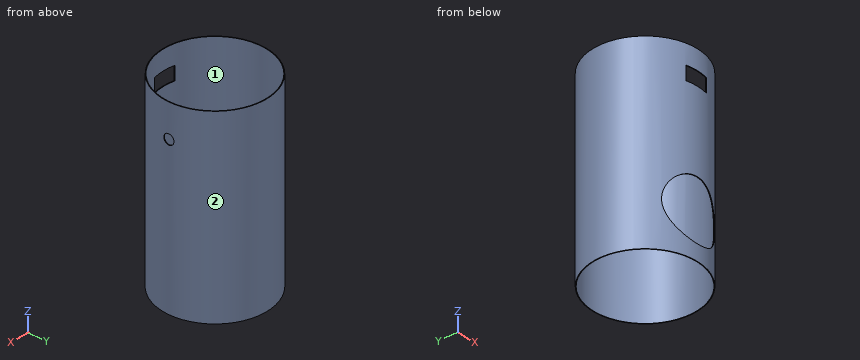
Autodesk Inventor part; units mm, degrees
ref_plane "WeldJoint" through (0, 0, -10) normal (0.5299, -0.848, 0) x (0, 0, 1)
ref_plane "Outer" through (0, 0, -10) normal (0.454, -0.891, 0) x (0, 0, 1)
ref_plane "Clock_Feeder" through (0, 0, -10) normal (0, 1, 0) x (0, 0, 1)
sketch "Sketch13" plane through (0, 0, 0) normal (0, 0, 1) x (1, 0, 0)
  circle A0 centre (0, 0) radius 470 construction
  line L0 (0, 0) -> (0, -470)
  line L1 (0, 0) -> (-398.5826, -249.0621)
  line L2 (0, 0) -> (470, 0)
  line L3 (0, 0) -> (0, -470)
  line L4 (0, 0) -> (0, -470)
  line L5 (0, 0) -> (-418.7731, -213.3755)
  arc A1 (-398.5826, -249.0621) -> (0, -470) centre (0, 0) ccw
  dimension "d53" = 940
  dimension "d54" = 58
  dimension "d55" = 0
  dimension "d56" = 0
  dimension "d57" = 270
  dimension "d58" = 63
ref_plane "WeldJoint" through (0, 0, -10) normal (0.5299, -0.848, 0) x (0, 0, 1)
ref_plane "Outer" through (0, 0, -10) normal (0.454, -0.891, 0) x (0, 0, 1)
ref_plane "Clock_Feeder" through (0, 0, -10) normal (0, 1, 0) x (0, 0, 1)
ref_plane "Charging" through (0, 0, -10) normal (1, 0, 0) x (0, 0, 1)
ref_plane "Accsess" through (0, 0, -10) normal (1, 0, 0) x (0, 0, 1)
sketch "Sketch14" plane through (0, 0, -10) normal (0.5299, -0.848, 0) x (0, 0, 1)
  line L0 (1710, 464) -> (10, 464)
  line L1 (10, 464) -> (10, 470)
  line L2 (10, 470) -> (1710, 470)
  line L3 (1710, 470) -> (1710, 464)
  line L4 (10, 0) -> (825.0673, 0)
  point P0 (10, 467)
  dimension "d59" = 1700
  dimension "d60" = 6
  dimension "d61" = 940
revolve "Revolution2" add sketch "Sketch14" angle 359.9 about axis through (0, 0, 0) along (0, 0, 1)
sketch "Sketch AnglePlane_Feeder" plane through (0, 0, -10) normal (0, 1, 0) x (0, 0, 1)
  line L0 (10, -470) -> (10, 470)
  line L1 (10, 0) -> (1410, 0)
  line L2 (1410, 0) -> (1410, 470)
  line L3 (1410, 470) -> (10, 470)
  line L4 (10, 470) -> (10, 0)
  point P0 (10, -398.5826)
  point P1 (10, -399.0167)
  dimension "d63" = 940
  dimension "d64" = 90
  dimension "frd_hght" = 1400
ref_plane "AnglePlane_Feeder" through (0, 0, 1400) normal (1, 0, 0) x (0, 1, 0)
sketch "Sketch16" plane through (0, 0, 1400) normal (1, 0, 0) x (0, 1, 0)
  circle A0 centre (0, 0) radius 45.5
  point P0 (0, -1400)
  point P1 (0, 0)
  point P2 (0, 0)
  point P3 (0, 0)
  dimension "d66" = 91
extrude "Extrusion7" cut sketch "Sketch16" along normal through all
ref_plane "Work Plane16" through (0, 0, 0) normal (0, -1, 0) x (1, 0, 0)
sketch "Sketch17" plane through (0, 0, 0) normal (0, -1, 0) x (1, 0, 0)
  circle A0 centre (0, 408.5) radius 268.5
  line L0 (0, 140) -> (-495.5727, 140)
  point P0 (0, 0)
  dimension "d69" = 537
  dimension "d71" = 140
extrude "Extrusion8" cut sketch "Sketch17" along normal through all
sketch "Sketch19" plane through (0, 0, -10) normal (1, 0, 0) x (0, 0, 1)
  line L0 (10, 0) -> (1410, 0)
  line L1 (1410, 0) -> (1410, 470)
  line L2 (1410, 470) -> (10, 470)
  line L3 (10, 470) -> (10, 0)
  dimension "d74" = 1400
  dimension "d76" = 940
  dimension "d77" = 90
ref_plane "Work Plane18" through (0, 0, 1400) normal (0, -1, 0) x (1, 0, 0)
sketch "Sketch20" plane through (0, 0, 1400) normal (0, -1, 0) x (1, 0, 0)
  line L0 (-103.5, 0) -> (103.5, 0)
  line L1 (103.5, 0) -> (103.5, 125)
  line L2 (103.5, 125) -> (-103.5, 125)
  line L3 (-103.5, 125) -> (-103.5, 0)
  point P0 (0, -1400)
  point P1 (0, 0)
  point P2 (0, 0)
  point P3 (0, 0)
  point P4 (0, 0)
  dimension "d78" = 207
  dimension "d79" = 125
extrude "Extrusion9" cut sketch "Sketch20" along normal through all
equation "\"BendRadius\" = Thickness"
equation "\"BendReliefWidth\" = Thickness"
equation "\"BendReliefDepth\" = 0.5 * Thickness"
equation "\"CornerReliefSize\" = 4 * Thickness"
equation "\"MinimumRemnant\" = 2 * Thickness"
equation "\"TransitionRadius\" = BendRadius"
equation "\"JacobiRadiusSize\" = BendRadius"
equation "\"GapSize\" = Thickness"
equation "\"Feeder_horisont_angle\" = 0"
equation "\"Hatch_Accsess_diameter\" = 535"
equation "\"Clock_Accsess_angle\" = 0"
equation "\"Clock_Charging_agnle\" = 0"
equation "\"Clock_Feeder_angle\" = 270deg"
equation "\"Clock_Outer_angle\" = 63deg"
equation "\"Clock_WeldJoint_angle\" = 58deg"
properties part number "PRS 940-10 main Shell D 940" material "Steel"
Here's how the part is built. I have some questions about the finished solid (model axes, mm). Face numbers are marked on the shaded views. Round coordinates to 2 decimals unless told otherwise and drop trailing zeros. Order: outer loops, then holes, each group sorted by start corner. A loop starts at its lowest first (then second) coordinate and runs counter-clockwise, first axis right, second up. Notation, with made-up numbers: (24, 12) -> (32, 12) arc R32 cw to (32, 38) -> close; hole circle Ø2 at (-31.75, 38.25). An arc over 180 degrees is marked (long way). Return JSON: item names as keys, results as strings.
Q1. I need wall thicknesses on line 1 along X through (y, z) = (15.5, 1578); line 2 along X through (y, z) = (7, 75); line 3 along Y through (x, z) = (380, 909). Which ranges of each line are inside material? Lowest first, please. Write a range as from..to.
Filled sheet:
{"line 1": "x = -469.74..-463.74, 463.74..469.74", "line 2": "x = -469.95..-463.95, 463.95..469.95", "line 3": "y = -276.59..-266.26, 266.26..276.59"}
Q2. For pin 1 Ø3 at (x, z) = (-276.5, 1014) entering from +Y; pin 2 Ø3 at (x, z) = (-118, 1513.5) entering from +Y; pin 3 Ø6 at (x, z) = (-50, 1303.5) entering from -Y; pin 4 Ø9 at (x, y) = (11, -462.5) entering from +Z, each with a flat end and sliding along its axis, tell me the tip position at first contact or that it passes through.
Filled sheet:
{"pin 1": "stops at y = 381.15", "pin 2": "stops at y = 455.33", "pin 3": "stops at y = -467.64", "pin 4": "stops at z = 1700"}
Q3. If we section it at D-D on z = 657: List the corners of the cut face in (x, y) for me.
Filled sheet:
{"outline": "(-399.02, -248.37) -> (-393.92, -245.2) arc R464 cw (long way) to (101.69, -452.72) -> (101.69, -458.87) arc R470 ccw (long way) to start; (-398.58, -249.06) arc R470 ccw to (-101.69, -458.87) -> (-101.69, -452.72) arc R464 cw to (-393.49, -245.88) -> close"}
Q4. If we section it at C-C on x = 205: List the corners of the cut face in (y, z) for me, plus the area to 3 significant figures.
Filled sheet:
{"outline": "(-422.94, 0) -> (-416.26, 0) -> (-416.26, 235.1) -> (-422.94, 235.1) -> close; (-422.94, 581.9) -> (-416.26, 581.9) -> (-416.26, 1700) -> (-422.94, 1700) -> close; (416.26, 0) -> (422.94, 0) -> (422.94, 1700) -> (416.26, 1700) -> close", "area": "20,400 mm^2"}
Q5. If we section it at B-B on y = 0: List the corners of the cut face in (x, z) for me.
Filled sheet:
{"outline": "(-470, 0) -> (-464, 0) -> (-464, 1700) -> (-470, 1700) -> close; (464, 0) -> (470, 0) -> (470, 1354.5) -> (464, 1354.5) -> close; (464, 1445.5) -> (470, 1445.5) -> (470, 1700) -> (464, 1700) -> close"}
Q6. If we mould it in two halves opening along Y, with no side actions, what happens to the marked faces 1 and 2? For each: released by +Y, released by -Y, zero draft, split by the parting line, or undercut.
Filled sheet:
{"face 1": "undercut", "face 2": "split by the parting line"}
Q7. If we section it at A-A on x = 0: List the corners of the cut face in (y, z) for me, plus the area to 3 significant figures.
Filled sheet:
{"outline": "(-470, 0) -> (-464, 0) -> (-464, 140) -> (-470, 140) -> close; (-470, 677) -> (-464, 677) -> (-464, 1400) -> (-470, 1400) -> close; (-470, 1525) -> (-464, 1525) -> (-464, 1700) -> (-470, 1700) -> close; (464, 0) -> (470, 0) -> (470, 1700) -> (464, 1700) -> close", "area": "16,400 mm^2"}
